The model under review builds one solid part; all positions refer to its coordinate system, in mm. Coordinates: 2 decimals unless noted, no trailing zeros. Order: outer loops, then holes, each group sorted by start corner. A loop starts at its lowest first (then second) coordinate and runs counter-clockwise, first axis right, second up. Notation, with made-up numbers: (28, 34.5) -> (83, 34.5) arc R19 cw to (83, 54.5) -> close; hole circle Ø2 at (25.5, 12.25). An arc over 180 degrees is marked (long way). Use one line per item in the form item = value. Start each with the question number.
(1) Insertion check: pin 1 Ø3 at (x, y) = (3, -3) entering from -Z. The pin has a flat end and moves straight along its axis. Give the tip position at first contact, or say it passes through.
(2) Mouldability with a two-part tool opening along X and no side actions: class faces 1 (the cylindrical face through (13.1, -5.14, 2.03)), 2 (the flat face through (7, -3, 4)), 3 (the cylindrical face through (0.86, -0.9, 2.03)), 4 (the cylindrical face through (9.55, -2.94, 1.97)) as +X half, -X half, draft (parallel to the pull), parting line (faces both ways), or undercut.
(3) Take a section at C-C (y = -1.7). State the section outline as (x, z) points.
(4) Take a section at A-A (z = 2.9). State how many separate pieces and enclosed holes the cut face has, then the cut area to 3 significant figures.
(5) Wall thickness on line 1 along Y through (x, z) = (11, 2.65); line 2 along Y through (x, z) = (3, 2.4); line 3 along X through (y, z) = (-1.9, 3.05): over which ranges is each line inside the solid? List them lowest first.
(6) Take a section at B-B (x = 10.25). State the section outline as (y, z) points.
(7) Take a section at D-D (y = -5.3). State the section outline as (x, z) points.
```python
from build123d import *

# Parameters (mm, degrees)
SKETCH1_W               = 14
SKETCH1_H               = 6
BOSS_EXTRUDE1_DEPTH     = 4
CUT_EXTRUDE1_DEPTH      = 16.748015748
CUT_EXTRUDE1_DEPTH_BACK = 16.748015748
SKETCH2_R               = 0.9
SKETCH2_R_2             = 1.45
FILLET1_R               = 3


with BuildPart() as part:
    # Sketch1 → Boss-Extrude1 (new body)
    with BuildSketch(Plane.XY):
        with Locations((7, -3)):
            Rectangle(SKETCH1_W, SKETCH1_H)
    extrude(amount=BOSS_EXTRUDE1_DEPTH)

    # Sketch2 → Cut-Extrude1 (cut, two sides: drawn at the far end of the back side and taken through both)
    with BuildSketch(Plane.XY.offset(4).offset(-CUT_EXTRUDE1_DEPTH_BACK)):
        with Locations((3, -3)):
            Circle(SKETCH2_R)
        with Locations((11, -3)):
            Circle(SKETCH2_R_2)
    extrude(amount=CUT_EXTRUDE1_DEPTH + CUT_EXTRUDE1_DEPTH_BACK, mode=Mode.SUBTRACT)

    # Fillet1
    fillet1_edges = [part.edges().sort_by_distance(p)[0] for p in [
        (14, -6, 2),
        (14, 0, 2),
        (0, -6, 2),
        (0, 0, 2),
    ]]
    fillet(fillet1_edges, radius=FILLET1_R - 0.0001)  # a hair under: the kernel refuses the full size


solid = part.part
```
Findings:
q1.pin_1 = 0
q2.face_1 = +X half
q2.face_2 = draft
q2.face_3 = -X half
q2.face_4 = undercut
q3.outline = (0.3, 0) -> (10.36, 0) -> (10.36, 4) -> (0.3, 4) -> close; (11.64, 0) -> (13.7, 0) -> (13.7, 4) -> (11.64, 4) -> close
q4.separate_pieces = 1
q4.enclosed_holes = 2
q4.area = 67.1 mm²
q5.line_1 = -6 to -4.45, -1.55 to 0
q5.line_2 = -6 to -3.9, -2.1 to 0
q5.line_3 = 0.21 to 10.06, 11.94 to 13.79
q6.outline = (-6, 0) -> (-4.24, 0) -> (-4.24, 4) -> (-6, 4) -> close; (-1.76, 0) -> (0, 0) -> (0, 4) -> (-1.76, 4) -> close
q7.outline = (1.07, 0) -> (12.93, 0) -> (12.93, 4) -> (1.07, 4) -> close
